Model file for the job. Use its own axes, mm. A direction names the side the tool comes from. Coordinates: 2 decimals unless noted, no trailing zeros. Write each loop counter-clockwise with the first axis right and the second up, starting at its lowest first coordinate (ties: lowest second). Pieces come first, ordered by that corner, then holes.
Q1. Pin check, flat tips, straight feed: P1, Ø4, axis at x = 3.5, y = -3.5, coming from the -Z side; P2, Ø2.5, axis at y = 1, z = 0.5, coming from the -X side; P3, Ø6, axis at x = 21.5, y = -1, coming from the -Z side. Stop position of each tip, or through.
Q2. Band-saw the part on A-A, the plane x = 8.5. Write the cut outline in (y, z), plus the area to 3 significant figures.
Q3. Drill centre lines: probe 1 along X at (y, z) = (-0.25, 4); probe 2 along Z at (x, y) = (2, 1); probe 3 along Z at (x, y) = (10, 2.75). Where is each one in solid material? Low to high.
Q4. Which spindle directions (+Z, -Z, +X, -X, +Y, -Y) get a long thin tool onto all of the face, cutting with end or side? Do faces 4 (the flat face through (24, 0, 0)), 5 (the flat face through (6, 3.3, -0.1)), 6 (the flat face through (1.479, 2.175, 1.233)). Say none if no direction does.
Q5. Pull direction Z, two halves, no side cores. Call faces 1 (the flat face through (1, 0, -2.5)), 2 (the flat face through (0, 2, 2)), 3 (the cylindrical face through (15, -3, 0)): released by +Z, released by -Z, zero draft, split by the parting line, or undercut.
Solid Edge part; units mm, degrees
sketch "Sketch1" plane through (0, 0, 0) normal (0, 0, 1) x (1, 0, 0)
  line L0 (0, 0) -> (0, 4.5)
  arc A0 (0, 4.5) -> (0.5, 5) centre (0.5, 4.5) cw
  line L1 (0.5, 5) -> (6, 5)
  line L2 (6, 5) -> (6, 3)
  line L3 (6, 3) -> (23.3865, 3)
  line L4 (23.3865, 3) -> (24, 2.3865)
  line L5 (24, 2.3865) -> (24, 0)
  line L6 (24, 0) -> (0, 0)
revolve "RevolvedProtrusion1" add sketch "Sketch1" angle 360 about axis through (24, 0, 0) along (-1, 0, 0)
cosmetic_thread "Thread1"
sketch "Sketch2" plane through (0, 0, 0) normal (1, 0, 0) x (0, 1, 0)
  line L0 (-1.4434, 2.5) -> (-2.8868, 0)
  line L1 (-2.8868, 0) -> (-1.4434, -2.5)
  line L2 (-1.4434, -2.5) -> (1.4434, -2.5)
  line L3 (1.4434, -2.5) -> (2.8868, 0)
  line L4 (2.8868, 0) -> (1.4434, 2.5)
  line L5 (1.4434, 2.5) -> (-1.4434, 2.5)
extrude "Cutout1" cut sketch "Sketch2" along normal blind 3
sketch "Sketch3" plane through (0, 0, 0) normal (0, 0, 1) x (1, 0, 0)
  line L0 (3, 0) -> (3, 2.5)
  line L1 (3, 2.5) -> (4.4434, 0)
  line L2 (4.4434, 0) -> (3, 0)
revolve "RevolvedCutout1" cut sketch "Sketch3" angle 360 about axis through (4.4434, 0, 0) along (-1, 0, 0)
properties part number "07160-206X18"
Answer sheet:
1. P1: stops at z = -4.77
1. P2: stops at x = 3.08
1. P3: stops at z = -3
2. outline: circle Ø6 at (0, 0)
2. area: 28.3 mm2
3. probe 1: x = 0 to 6
3. probe 2: z = -4.9 to -2.5, 2.5 to 4.9
3. probe 3: z = -1.2 to 1.2
4. face 4: +Z, -Z, +X, +Y, -Y
4. face 5: +X
4. face 6: -X
5. face 1: undercut
5. face 2: zero draft
5. face 3: split by the parting line
